CAD build for the part. Positions are in the model's coordinates, mm. Face numbers are marked on the shaded views. A direction names the side the tool comes from. Give positions to 0.01 mm unless a question says otherwise; leave off trailing zeros. Write each loop counter-clockwise with the first axis right and the second up, starting at its lowest first coordinate (ties: lowest second). Pieces come first, ordered by that corner, then holes. Notation, with made-up numbers: (25.5, 77) - (31.5, 77) arc R26 cw to (31.5, 103) - close; hole circle Ø10 at (-25, -25). An arc over 180 degrees is marked (long way). Put each result on its own line as item: value. Start each with the question number.
1. Mould opens along X. For the marked faces 1, 2, 3 and 4 say: +X half, -X half, draft (parallel to the pull), parting line (faces both ways), or undercut.
2. Wall check: line 1 (X direction, y = 64.5, z = 0); line 2 (Z direction, x = 29.5, y = 0.7); line 3 (Z direction, x = -2, y = 73). Give the ranges that are in metal, low to high.
3. Cut at D-D on z = -27.5. List the corners of the cut face in (x, y), and give its area (3 significant figures).
4. Drop flat-ended pins along their axis: pin 1 (5 mm diameter, centred on x = -14.5, z = 9, fed in from +Y); pin 2 (5 mm diameter, centred on x = -29.5, z = 34, fed in from +Y); pin 3 (15.5 mm diameter, centred on x = -19.5, y = 49.5, fed in from +Z). Give the stop position or say it passes through.
5. Tool access for the marked faces 5 and 6: list every direction of +Z, -Z, +X, -X, +Y, -Y with a clear straight run to the whole face (end or side of a thin tool).
6. Cut at C-C on x = 23. List the corners of the cut face in (y, z), and give its area (3 significant figures).
7. Cut at A-A on z = 35. List the corners of the cut face in (x, y), and give its area (3 significant figures).
8. Cut at B-B on y = 58. List the corners of the cut face in (x, z).
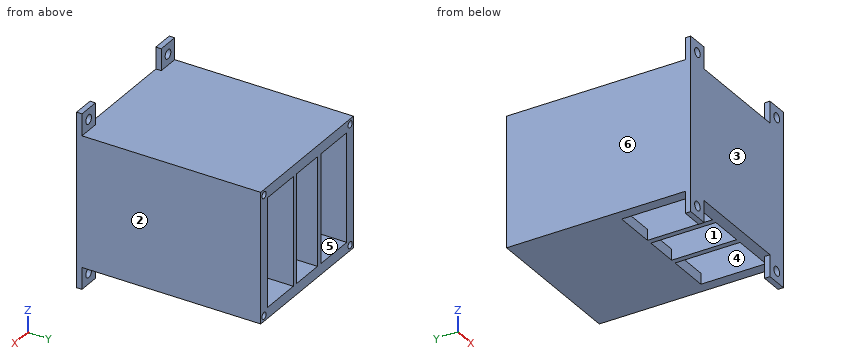
Autodesk Inventor part; units mm, degrees
ref_plane "Work Plane2" through (-34.5, 85, 0) normal (0, 0, 1) x (1, 0, 0)
ref_plane "Work Plane3" through (0, 85, 25) normal (1, 0, 0) x (0, 0, -1)
ref_plane "YZ Plane" through (0, 0, 0) normal (1, 0, 0) x (0, 1, 0)
sketch "Sketch1" plane through (0, 0, 0) normal (0, 1, 0) x (-1, 0, 0)
  point P0 (0, 0)
sketch "Sketch2" plane through (0, 0, 0) normal (0, 1, 0) x (-1, 0, 0)
  line L0 (34.5, 30) -> (-34.5, 30)
  line L1 (-34.5, 30) -> (-34.5, -30)
  line L2 (-34.5, -30) -> (34.5, -30)
  line L3 (34.5, -30) -> (34.5, 30)
  line L4 (34.5, 30) -> (-34.5, -30) construction
  line L5 (-34.5, 30) -> (34.5, -30) construction
  point P0 (0, 0)
  dimension "d0" = 69
  dimension "d1" = 60
extrude "Extrusion1" add sketch "Sketch2" along normal blind 85
sketch "Sketch3" plane through (0, 85, 0) normal (0, 1, 0) x (1, 0, 0)
  line L0 (-29.5, -25) -> (29.5, -25)
  line L1 (29.5, -25) -> (29.5, 25)
  line L2 (29.5, 25) -> (-29.5, 25)
  line L3 (-29.5, 25) -> (-29.5, -25)
  line L4 (-29.5, -25) -> (29.5, 25) construction
  line L5 (29.5, -25) -> (-29.5, 25) construction
  point P0 (0, 0)
  dimension "d4" = 59
  dimension "d5" = 50
extrude "Extrusion2" cut sketch "Sketch3" against normal blind 80
sketch "Sketch4" plane through (0, 85, 0) normal (0, 1, 0) x (1, 0, 0)
  circle A0 centre (32, -27.5) radius 1.55
  line L0 (-34.5, -30) -> (34.5, -30)
  line L1 (34.5, -30) -> (34.5, 30)
  circle A1 centre (32, 27.5) radius 1.55
  circle A2 centre (-32, 27.5) radius 1.55
  circle A3 centre (-32, -27.5) radius 1.55
  line L2 (34.5, 30) -> (-34.5, 30)
  line L3 (-34.5, 30) -> (-34.5, -30)
  point P0 (0, 0)
  dimension "d8" = 3.1
  dimension "d9" = 2.5
  dimension "d10" = 2.5
  dimension "d11" = 2.5
  dimension "d12" = 2.5
extrude "Extrusion3" cut sketch "Sketch4" against normal blind 10 contours A0 | A1 | A2 | A3
sketch "Sketch5" plane through (-34.5, 0, 30) normal (0, 0, 1) x (1, 0, 0)
  line L0 (0, 0) -> (0, 85)
  line L1 (0, 0) -> (10, 0)
  line L2 (10, 0) -> (10, 2.5)
  line L3 (10, 2.5) -> (0, 2.5)
  line L4 (0, 2.5) -> (0, 0)
  line L5 (34.5, 0) -> (34.5, 85)
  line L6 (5, 85) -> (64, 85)
  line L7 (69, 0) -> (59, 0)
  line L8 (59, 0) -> (59, 2.5)
  line L9 (59, 2.5) -> (69, 2.5)
  line L10 (69, 2.5) -> (69, 0)
  dimension "d15" = 10
  dimension "d16" = 2.5
extrude "Extrusion4" add sketch "Sketch5" along normal blind 10
sketch "Sketch6" plane through (-34.5, 2.5, 30) normal (0, 1, 0) x (1, 0, 0)
  circle A0 centre (5, -5) radius 2.1
  line L0 (10, -10) -> (0, -10)
  line L1 (0, 0) -> (0, -10)
  line L2 (69, 60) -> (0, 60)
  line L3 (34.5, 60) -> (34.5, 0)
  line L4 (0, 0) -> (69, 0)
  circle A1 centre (64, -5) radius 2.1
  point P0 (34.5, 30)
  dimension "d19" = 4.2
  dimension "d20" = 5
  dimension "d21" = 5
extrude "Extrusion5" cut sketch "Sketch6" against normal up to next
ref_plane "Work Plane2" through (-34.5, 85, 0) normal (0, 0, 1) x (1, 0, 0)
mirror "Mirror2" about plane through (-34.5, 85, 0) normal (0, 0, 1) of "Extrusion4", "Extrusion5"
sketch "Sketch7" plane through (34.5, 85, -30) normal (0, 0, -1) x (-1, 0, 0)
  line L0 (5, 0) -> (5, -80)
  line L1 (64, 0) -> (64, -80)
  line L2 (5, -80) -> (64, -80)
  line L3 (64, -80) -> (64, -50)
  line L4 (64, -50) -> (5, -50)
  line L5 (5, -50) -> (5, -80)
  point P0 (34.5, -85)
  point P1 (5, -50)
  dimension "d24" = 30
extrude "Extrusion6" cut sketch "Sketch7" against normal up to next
sketch "Sketch8" plane through (0, 5, 0) normal (0, 1, 0) x (1, 0, 0)
  line L0 (-29.5, 25) -> (29.5, 25)
  line L1 (-6.5, -25) -> (6.5, -25)
  line L2 (6.5, -25) -> (6.5, 25)
  line L3 (6.5, 25) -> (-6.5, 25)
  line L4 (-6.5, 25) -> (-6.5, -25)
  line L5 (-6.5, -25) -> (6.5, 25) construction
  line L6 (6.5, -25) -> (-6.5, 25) construction
  line L7 (29.5, -25) -> (-29.5, -25)
  line L8 (-6.5, 25) -> (-11.5, 25)
  line L9 (-11.5, 25) -> (-11.5, -25)
  line L10 (-11.5, -25) -> (-6.5, -25)
  line L11 (-6.5, -25) -> (-6.5, 25)
  line L12 (6.5, -25) -> (11.5, -25)
  line L13 (11.5, -25) -> (11.5, 25)
  line L14 (11.5, 25) -> (6.5, 25)
  line L15 (6.5, 25) -> (6.5, -25)
  line L16 (-10.25, 25) -> (-7.75, 25)
  line L17 (-7.75, 25) -> (-7.75, -26.1279)
  line L18 (-7.75, -26.1279) -> (-10.25, -26.1279)
  line L19 (-10.25, -26.1279) -> (-10.25, 25)
  point P0 (0, 0)
  point P1 (-10.25, -25)
  point P2 (-7.75, -25)
  dimension "d27" = 13
  dimension "d28" = 5
  dimension "d29" = 5
  dimension "d30" = 1.25
  dimension "d31" = 1.25
extrude "Extrusion7" add sketch "Sketch8" along normal blind 80 contours L0 L17 L7 L19
ref_plane "Work Plane3" through (0, 85, 25) normal (1, 0, 0) x (0, 0, -1)
mirror "Mirror3" about plane through (0, 85, 25) normal (1, 0, 0) of "Extrusion7"
sketch "Sketch9" plane through (10.25, 35, -25) normal (0, 0, -1) x (-1, 0, 0)
  line L0 (0, -30) -> (0, 50)
  line L1 (2.5, 0) -> (2.5, 50)
  line L2 (0, -30) -> (2.5, -30)
  line L3 (2.5, -30) -> (2.5, 0)
  line L4 (2.5, 0) -> (0, 0)
  line L5 (0, 0) -> (0, -30)
  line L6 (18, -30) -> (18, 0)
  line L7 (20.5, 50) -> (20.5, -30)
  line L8 (18, -30) -> (20.5, -30)
  line L9 (20.5, -30) -> (20.5, 0)
  line L10 (20.5, 0) -> (18, 0)
  line L11 (18, 0) -> (18, -30)
  point P0 (10.25, -35)
extrude "Extrusion8" add sketch "Sketch9" along normal blind 5
equation "\"d0\" = external_len"
equation "\"d1\" = external_width"
equation "\"d2\" = internal_height + thickness"
equation "\"d4\" = internal_len"
equation "\"d5\" = internal_width"
equation "\"d6\" = internal_height"
equation "\"d32\" = internal_height"
equation "\"d34\" = thickness"
equation "\"external_len\" = 69"
equation "\"external_width\" = 60"
equation "\"thickness\" = 5"
equation "\"internal_height\" = 80"
equation "\"separator_thickness\" = 2.5"
equation "\"switch_len_at_clip\" = 13"
equation "\"internal_len\" = external_len - 2 * thickness"
equation "\"internal_width\" = external_width - 2 * thickness"
properties part number "switch_pannel_box"
Report:
1. face 1: undercut
1. face 2: +X half
1. face 3: draft
1. face 4: undercut
2. line 1: x = -34.5 to -29.5, -10.25 to -7.75, 7.75 to 10.25, 29.5 to 34.5
2. line 2: z = -40 to -37.1, -32.9 to 32.9, 37.1 to 40
2. line 3: z = -30 to -25, 25 to 30
3. outline: (-34.5, 0) - (34.5, 0) - (34.5, 85) - (33.55, 85) - (33.55, 75) - (30.45, 75) - (30.45, 85) - (-30.45, 85) - (-30.45, 75) - (-33.55, 75) - (-33.55, 85) - (-34.5, 85) - close; hole (-29.5, 5) - (-10.25, 5) - (-10.25, 35) - (-29.5, 35) - close; hole (-7.75, 5) - (7.75, 5) - (7.75, 35) - (-7.75, 35) - close; hole (10.25, 5) - (29.5, 5) - (29.5, 35) - (10.25, 35) - close
3. area: 4,180 mm²
4. pin 1: stops at y = 5
4. pin 2: stops at y = 2.5
4. pin 3: stops at z = 30
5. face 5: +Y
5. face 6: +Z, -Z, -X, +Y, -Y
6. outline: (0, -30) - (5, -30) - (5, 25) - (85, 25) - (85, 30) - (0, 30) - close; (35, -30) - (85, -30) - (85, -25) - (35, -25) - close
6. area: 950 mm²
7. outline: (-34.5, 0) - (-31.6, 0) - (-31.6, 2.5) - (-34.5, 2.5) - close; (-27.4, 0) - (-24.5, 0) - (-24.5, 2.5) - (-27.4, 2.5) - close; (24.5, 0) - (27.4, 0) - (27.4, 2.5) - (24.5, 2.5) - close; (31.6, 0) - (34.5, 0) - (34.5, 2.5) - (31.6, 2.5) - close
7. area: 29.0 mm²
8. outline: (-34.5, -30) - (34.5, -30) - (34.5, 30) - (-34.5, 30) - close; hole (-29.5, -25) - (-10.25, -25) - (-10.25, 25) - (-29.5, 25) - close; hole (-7.75, -25) - (7.75, -25) - (7.75, 25) - (-7.75, 25) - close; hole (10.25, -25) - (29.5, -25) - (29.5, 25) - (10.25, 25) - close
